Geometry: final body of the model. Coordinates: model frame, mm. Round coordinates to 2 decimals unless told otherwise and drop trailing zeros. Order: outer loops, then holes, each group sorted by start corner. A loop starts at its lowest first (then second) coordinate and runs counter-clockwise, first axis right, second up. Notation, with made-up numbers: M 76.25,77.5 L 127.25,77.5 A22 ccw 127.25,98.5 Z; hole C 34,66 d11. An arc over 180 degrees is marked long. Return JSON: item names as keys, results as strings. Group by question number.
Q1. Cut plane C-C on x = 220. Output: boundary loops of the cut face in (y, z).
Q2. Cut plane D-D on z = 91. Output: boundary loops of the cut face in (x, y).
Q3. Cut plane A-A on z = 26. Output: boundary loops of the cut face in (x, y).
Q4. Contact query for a flat-ended pin moving along its axis: pin 1 (1 mm diameter, centred on y = -3.5, z = 156, fed in from +X). Output: stop coordinate, or through.
Q5. Cut plane B-B on y = -2.1. Output: boundary loops of the cut face in (x, z).
Q6. Ray query, probe 1 along Z at (x, y) = (315.5, -2.6); probe 2 along X at (y, z) = (-2.45, 34); probe 3 along X at (y, z) = (-3.25, 31). Return the intervals inside material, ascending.
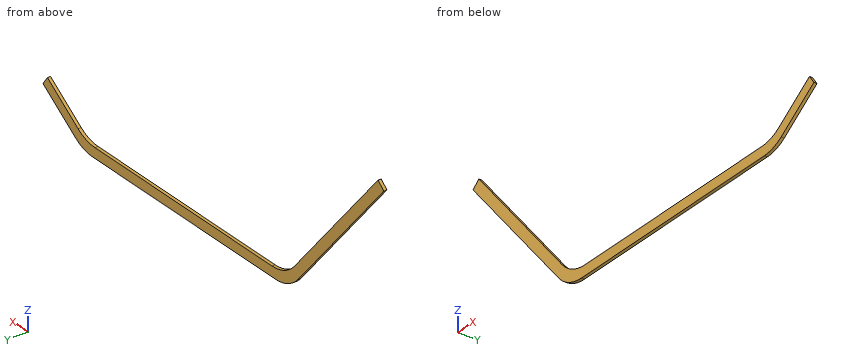
```python
from build123d import *

# Parameters (mm, degrees)
F1_DEPTH = 4


with BuildPart() as f1:
    # F0 (on Front) → F1 (new body)
    with BuildSketch(Plane.XZ):
        with BuildLine():
            ThreePointArc((-26.156867, 4.884096), (-8.985558, -8.291913), (12.145355, -12.976524))
            Line((12.145355, -12.976524), (323.065033, -12.976524))
            ThreePointArc((323.065033, -12.976524), (338.100323, -10.662371), (351.743855, -3.934126))
            Line((351.743855, -3.934126), (407.221116, 34.911471))
            Line((407.221116, 34.911471), (399.764622, 45.560447))
            Line((399.764622, 45.560447), (347.64497, 9.065874))
            ThreePointArc((347.64497, 9.065874), (334.001439, 2.337629), (318.966149, 0.023476))
            Line((318.966149, 0.023476), (18.207355, 0.023476))
            ThreePointArc((18.207355, 0.023476), (-2.923558, 4.708087), (-20.094867, 17.884096))
            Line((-20.094867, 17.884096), (-161.908352, 186.890826))
            Line((-161.908352, 186.890826), (-171.86693, 178.534587))
            Line((-171.86693, 178.534587), (-26.156867, 4.884096))
        make_face()
    extrude(amount=F1_DEPTH)


solid = f1.part
```
Result sheet:
{
 "1": {"outline": "M -4,-12.98 L 0,-12.98 L 0,0.02 L -4,0.02 Z"},
 "2": {"outline": "M -98.42,-4 L -81.45,-4 L -81.45,0 L -98.42,0 Z"},
 "3": {"outline": "M -43.88,-4 L -26.9,-4 L -26.9,0 L -43.88,0 Z; M 371.83,-4 L 394.49,-4 L 394.49,0 L 371.83,0 Z"},
 "4": {"pin 1": "stops at x = -135.57"},
 "5": {"outline": "M -171.87,178.53 L -26.16,4.88 A50 ccw 12.15,-12.98 L 323.07,-12.98 A50 ccw 351.74,-3.93 L 407.22,34.91 L 399.76,45.56 L 347.64,9.07 A50 cw 318.97,0.02 L 18.21,0.02 A50 cw -20.09,17.88 L -161.91,186.89 Z"},
 "6": {"probe 1": "z = -12.98 to 0.02", "probe 2": "x = -50.59 to -33.62, 383.25 to 405.92", "probe 3": "x = -48.07 to -31.1, 378.97 to 401.63"}
}
